Model file for the job. Use its own axes, mm. A direction names the side the tool comes from. Round coordinates to 2 decimals unless told otherwise and drop trailing zeros. Loops run counter-clockwise (first coordinate to the right, second up) from the corner with the lowest first, then second, coordinate; pieces in that order, holes last. Notation, with made-up numbers: (74.25, -20.75) - (99.25, -20.75) arc R18 cw to (99.25, 8.25) - close; hole circle Ø10 at (4, 31.5). An arc over 180 degrees is marked (long way). Answer as a JSON object with one key per item and string values.
Autodesk Inventor part; units mm, degrees
ref_plane "YZ Plane" through (0, 0, 0) normal (1, 0, 0) x (0, 1, 0)
ref_plane "XZ Plane" through (0, 0, 0) normal (0, 1, 0) x (-1, 0, 0)
ref_plane "XY Plane" through (0, 0, 0) normal (0, 0, 1) x (1, 0, 0)
sketch "Skizze1" plane through (0, 0, 0) normal (0, 0, 1) x (1, 0, 0)
  line L0 (0, 0) -> (2.7641, 0)
  line L1 (6, 6) -> (6, 80)
  line L2 (6, 80) -> (0, 80)
  line L3 (0, 80) -> (0, 0)
  line L4 (-8, 0) -> (48, 0)
  line L5 (0, -16) -> (0, 96)
  line L6 (0, 0) -> (40, 0)
  line L7 (40, 0) -> (40, 6)
  line L8 (40, 6) -> (6, 6)
  line L9 (0, 2.8256) -> (0, 0)
  dimension "d0" = 80
  dimension "d1" = 40
  dimension "d2" = 6
extrude "Extrusion1" add sketch "Skizze1" along normal blind 40
sketch "Skizze2" plane through (6, 6, 0) normal (0, 1, 0) x (1, 0, 0)
  line L0 (34, 0) -> (34, -40)
  line L1 (0, 0) -> (0, -40)
  line L2 (0, -20) -> (34, -20)
  line L3 (0, -7.5) -> (34, -7.5)
  line L4 (34, -7.5) -> (34, -32.5)
  line L5 (34, -32.5) -> (0, -32.5)
  line L6 (0, -32.5) -> (0, -7.5)
  line L7 (34, -7.5) -> (0, -7.5)
  line L8 (0, -7.5) -> (0, 0)
  line L9 (0, 0) -> (34, 0)
  line L10 (34, 0) -> (34, -7.5)
  line L11 (34, -40) -> (0, -40)
  line L12 (0, -40) -> (0, -32.5)
  line L13 (0, -32.5) -> (34, -32.5)
  line L14 (34, -32.5) -> (34, -40)
  point P0 (-6, 0)
  dimension "d5" = 25
extrude "Extrusion2" cut sketch "Skizze2" against normal through all contours L0 L3 L1 L9 | L0 L11 L1 L5
sketch "Skizze3" plane through (0, 0, 0) normal (-1, 0, 0) x (0, 0, 1)
  line L0 (0, 80) -> (40, 80)
  line L1 (0, 0) -> (40, 0)
  line L2 (20, 80) -> (20, 0)
  point P0 (20, 65)
  point P1 (20, 35)
  dimension "d8" = 15
  dimension "d9" = 30
hole "Bohrung1" at (0, 65, 20) at (0, 35, 20) direction (1, 0, 0) diameter 4 end through all
sketch "Skizze4" plane through (6, 6, 32.5) normal (0, 1, 0) x (1, 0, 0)
  line L0 (34, 25) -> (34, 0)
  line L1 (0, 25) -> (0, 0)
  line L2 (34, 12.5) -> (0, 12.5)
  point P0 (-6, 32.5)
  point P1 (29, 12.5)
  point P2 (9, 12.5)
  dimension "d17" = 20
  dimension "d59" = 5
hole "Bohrung2" at (35, 6, 20) at (15, 6, 20) direction (0, -1, 0) diameter 4.5 end through all
sketch "Skizze5" plane through (0, 0, 0) normal (0, -1, 0) x (1, 0, 0)
  circle A0 centre (15, 20) radius 2.25
  circle A1 centre (35, 20) radius 2.25
  line L0 (40, 32.5) -> (6, 32.5)
  line L1 (6, 32.5) -> (6, 7.5)
  line L2 (15, 20) -> (35, 20)
  line L3 (40, 7.5) -> (40, 32.5)
  line L4 (25, 20) -> (25, 16.5238)
  dimension "d60" = 10
  dimension "d61" = 10
hole "Bohrung4" at (25, 0, 20) direction (0, 1, 0) diameter 5.1 end through all
fillet "Rundung1" radius 5 2 edges at (6, 3, 7.5) (6, 3, 32.5)
sketch "Skizze7" plane through (6, 0, 0) normal (1, 0, 0) x (0, 0, -1)
  circle A0 centre (-20, 65) radius 2
  circle A1 centre (-20, 35) radius 2
hole "Bohrung7" at (6, 65, 20) at (6, 35, 20) direction (-1, 0, 0) diameter 4.5 end through all countersink diameter 9.2 countersink angle 90
properties part number "1_0204_006"
1) Two-plate mould, pull along X, no slides. Class faces 4 (the cylindrical face through (1.799, 67.196, 20.488)), 5 (the flat face through (6, 39, 15)), 6 (the flat face through (0, 41, 20)), 7 (the cylindrical face through (33.103, 2.958, 21.21)): pulls with the +X half, pulls with the -X half, needs draft (parallel to the pull), parting line crosses it, or undercut.
Values follow:
{"face 4": "needs draft", "face 5": "pulls with the +X half", "face 6": "pulls with the -X half", "face 7": "undercut"}
2) Slice it at D-D on x = 5. List the corners of the cut face in (y, z), then the cut area to 3 significant figures.
Values follow:
{"outline": "(0, 0) - (80, 0) - (80, 40) - (0, 40) - close; hole circle Ø7.2 at (35, 20); hole circle Ø7.2 at (65, 20)", "area": "3,120 mm²"}
3) Slice it at C-C on x = 15. List the corners of the cut face in (y, z).
Values follow:
{"outline": "(0, 7.5) - (6, 7.5) - (6, 17.75) - (0, 17.75) - close; (0, 22.25) - (6, 22.25) - (6, 32.5) - (0, 32.5) - close"}
4) Drop flat-ended pins along their axis: P1, Ø4, axis at x = 13.5, z = 20.5, coming from the +Y side; P2, Ø2, axis at y = 44, z = 23.5, coming from the -X side; P3, Ø3, axis at y = 65.5, z = 18.5, coming from the +X side; P4, Ø6.5, axis at x = 25, y = 4, coming from the -Z side. Give the stop position or say it passes through.
Values follow:
{"P1": "y = 6", "P2": "x = 0", "P3": "x = 4.48", "P4": "z = 7.5"}
5) Probe probe 1 along X at (y, z) = (4, 20); probe 2 along Z at (x, y) = (25, 1); probe 3 along Z at (x, y) = (35, 2.15). List the from-to ranges inside material, lowest first.
Values follow:
{"probe 1": "0 to 12.75, 17.25 to 22.45, 27.55 to 32.75, 37.25 to 40", "probe 2": "7.5 to 17.45, 22.55 to 32.5", "probe 3": "7.5 to 17.75, 22.25 to 32.5"}
6) Slice it at A-A on y = 35. List the corners of the cut face in (x, z).
Values follow:
{"outline": "(0, 0) - (6, 0) - (6, 15.4) - (3.65, 17.75) - (0, 17.75) - close; (0, 22.25) - (3.65, 22.25) - (6, 24.6) - (6, 40) - (0, 40) - close"}
7) Slice it at B-B on z = 20. Count the separate pieces of the cut face and the enclosed holes in it, then the cut area to 3 significant figures.
Values follow:
{"separate pieces": "6", "enclosed holes": "0", "area": "534 mm²"}
8) Tool access for faces 1 (the flat face through (19, 6, 20)), 2 (the flat face through (26, 3, 32.5)), 3 (the flat face through (25, 3, 7.5)): list every direction of +Z, -Z, +X, -X, +Y, -Y with a clear straight run to the whole face (end or side of a thin tool).
Values follow:
{"face 1": "+Z, -Z, +X, +Y", "face 2": "+Z, +X, +Y, -Y", "face 3": "-Z, +X, +Y, -Y"}
